Can you work these out from the model? Positions are in its coordinate system, mm. Give positions to 0.01 mm unless a question says otherwise; leave off trailing zeros. Order: outer loops, then holes, each group sorted by start corner. A loop starts at its lowest first (then second) coordinate and runs counter-clockwise, first axis right, second up.
Item 1: I'm going to push a flat-ended pin straight in: pin 1 Ø2.5 at (x, y) = (45, 4) entering from -Z. Where does the tip first touch, or does it pass through?
Item 2: If I drill on line 1 along Z through (x, y) = (-5.5, 0.5); line 2 along Z through (x, y) = (23, 0.5), over which ranges is the centre line in solid material (lowest first)?
Item 3: I want a section at C-C, the plane z = 30.5. Write out the boundary of the cut face in (x, y), then the cut area to 3 significant figures.
Item 4: I want a section at A-A, the plane z = -45.5. Count the separate pieces of the cut face and the enclosed holes in it, then the cut area to 3 significant figures.
Item 5: I want a section at D-D, the plane z = 45.5. Write out the boundary of the cut face in (x, y), then the cut area to 3 significant figures.
Item 6: I want a section at B-B, the plane x = -3. Write out the boundary of the cut face in (y, z), then the cut area to 3 significant figures.
```python
from build123d import *

# Parameters (mm, degrees)
SKETCH1_W                       = 96
SKETCH1_H                       = 96
SKETCH1_W_2                     = 80
SKETCH1_H_2                     = 80
BOSS_EXTRUDE1_DEPTH             = 8
F_3_0_3_DIAMETER_HOLE6_D        = 3
F_3_0_3_DIAMETER_HOLE6_DEPTH    = 7.5
F_3_0_3_DIAMETER_HOLE3_D        = 3
F_3_0_3_DIAMETER_HOLE3_DEPTH    = 7.5
SKETCH27_W                      = 82
SKETCH27_H                      = 82
CUT_EXTRUDE2_DEPTH              = 10
F_3_4_3_4_DIAMETER_HOLE1_D      = 3.4
SKETCH38_W                      = 85
SKETCH38_H                      = 85
CUT_EXTRUDE4_DEPTH              = 10
SKETCH44_W                      = 4
SKETCH44_H                      = 4
BOSS_EXTRUDE2_DEPTH             = 8
SKETCH45_W                      = 4
SKETCH45_H                      = 3.5
BOSS_EXTRUDE3_DEPTH             = 8
TAP_DRILL_FOR_M3X0_5_TAP1_D     = 2.5
SKETCH49_W                      = 96
SKETCH49_H                      = 1.5
CUT_EXTRUDE5_DEPTH              = 146
TAP_DRILL_FOR_M3X0_5_TAP2_D     = 3
TAP_DRILL_FOR_M3X0_5_TAP2_DEPTH = 5.5
TAP_DRILL_FOR_M3X0_5_TAP3_D     = 3
TAP_DRILL_FOR_M3X0_5_TAP3_DEPTH = 5.5
TAP_DRILL_FOR_M3X0_5_TAP4_D     = 3
TAP_DRILL_FOR_M3X0_5_TAP5_D     = 3
TAP_DRILL_FOR_M3X0_5_TAP6_D     = 3
TAP_DRILL_FOR_M3X0_5_TAP6_DEPTH = 5.5


with BuildPart() as part:
    # Sketch1 → Boss-Extrude1 (new body)
    with BuildSketch(Plane(origin=(0, 0, 0), x_dir=(1, 0, 0), z_dir=(0, 1, 0))):
        Rectangle(SKETCH1_W, SKETCH1_H)
        Rectangle(SKETCH1_W_2, SKETCH1_H_2, mode=Mode.SUBTRACT)
    extrude(amount=BOSS_EXTRUDE1_DEPTH)

    # Ø3.0 (3) Diameter Hole6
    with Locations(Plane.XY.offset(48)):
        with Locations((45, 4), (-45, 4)):
            Hole(F_3_0_3_DIAMETER_HOLE6_D / 2, depth=F_3_0_3_DIAMETER_HOLE6_DEPTH)

    # Ø3.0 (3) Diameter Hole3
    with Locations(Plane(origin=(0, 0, -48), x_dir=(-1, 0, 0), z_dir=(0, 0, -1))):
        with Locations((-45, 4), (45, 4)):
            Hole(F_3_0_3_DIAMETER_HOLE3_D / 2, depth=F_3_0_3_DIAMETER_HOLE3_DEPTH)

    # Sketch27 → Cut-Extrude2 (cut)
    with BuildSketch(Plane(origin=(0, 8, 0), x_dir=(1, 0, 0), z_dir=(0, 1, 0))):
        Rectangle(SKETCH27_W, SKETCH27_H)
    extrude(amount=-CUT_EXTRUDE2_DEPTH, mode=Mode.SUBTRACT)

    # Ø3.4 (3.4) Diameter Hole1 (through all)
    with Locations(Plane(origin=(0, 0, 0), x_dir=(-1, 0, 0), z_dir=(0, -1, 0))):
        with Locations((-23, 45.5), (23, 45.5), (45.5, 23), (45.5, -25), (23, -45.5), (-23, -45.5), (-45.5, -25), (-45.5, 25)):
            Hole(F_3_4_3_4_DIAMETER_HOLE1_D / 2)

    # Sketch38 → Cut-Extrude4 (cut)
    with BuildSketch(Plane(origin=(0, 8, 0), x_dir=(1, 0, 0), z_dir=(0, 1, 0))):
        Rectangle(SKETCH38_W, SKETCH38_H)
    extrude(amount=-CUT_EXTRUDE4_DEPTH, mode=Mode.SUBTRACT)

    # Sketch44 → Boss-Extrude2 (add)
    with BuildSketch(Plane.XZ):
        with Locations((40.5, -40.5)):
            Rectangle(SKETCH44_W, SKETCH44_H)
        with Locations((-40.5, -40.5)):
            Rectangle(SKETCH44_W, SKETCH44_H)
        with Locations((-40.5, 40.5)):
            Rectangle(SKETCH44_W, SKETCH44_H)
        with Locations((40.5, 40.5)):
            Rectangle(SKETCH44_W, SKETCH44_H)
    extrude(amount=-BOSS_EXTRUDE2_DEPTH)

    # Sketch45 → Boss-Extrude3 (add)
    with BuildSketch(Plane(origin=(0, 8, 0), x_dir=(1, 0, 0), z_dir=(0, 1, 0))):
        with Locations((-40.5, 36.75)):
            Rectangle(SKETCH45_W, SKETCH45_H)
    extrude(amount=-BOSS_EXTRUDE3_DEPTH)

    # Tap Drill for M3x0.5 Tap1 (through all)
    with Locations(Plane(origin=(0, 8, 0), x_dir=(1, 0, 0), z_dir=(0, 1, 0))):
        with Locations((41.5, 41.5), (41.5, -41.5), (-41.5, -41.5), (-44.05, 37.33)):
            Hole(TAP_DRILL_FOR_M3X0_5_TAP1_D / 2)

    # Sketch49 → Cut-Extrude5 (cut)
    with BuildSketch(Plane(origin=(48, 0, 0), x_dir=(0, 0, -1), z_dir=(1, 0, 0))):
        with Locations((0, 7.25)):
            Rectangle(SKETCH49_W, SKETCH49_H)
    extrude(amount=-CUT_EXTRUDE5_DEPTH, mode=Mode.SUBTRACT)

    # Tap Drill for M3x0.5 Tap2
    with Locations(Plane.ZY.offset(48)):
        with Locations((30.5, 3.7), (-30.5, 3.7)):
            Hole(TAP_DRILL_FOR_M3X0_5_TAP2_D / 2, depth=TAP_DRILL_FOR_M3X0_5_TAP2_DEPTH)

    # Tap Drill for M3x0.5 Tap3
    with Locations(Plane(origin=(0, 0, -48), x_dir=(-1, 0, 0), z_dir=(0, 0, -1))):
        with Locations((30.5, 3.7), (-30.5, 3.7)):
            Hole(TAP_DRILL_FOR_M3X0_5_TAP3_D / 2, depth=TAP_DRILL_FOR_M3X0_5_TAP3_DEPTH)

    # Tap Drill for M3x0.5 Tap4 (through all)
    with Locations(Plane(origin=(48, 0, 0), x_dir=(0, 0, -1), z_dir=(1, 0, 0))):
        with Locations((30.5, 3.7), (-30.5, 3.7)):
            Hole(TAP_DRILL_FOR_M3X0_5_TAP4_D / 2)

    # Tap Drill for M3x0.5 Tap5 (through all)
    with Locations(Plane.XY.offset(48)):
        with Locations((30.5, 3.7), (-30.5, 3.7)):
            Hole(TAP_DRILL_FOR_M3X0_5_TAP5_D / 2)

    # Tap Drill for M3x0.5 Tap6
    with Locations(Plane(origin=(0, 0, -48), x_dir=(-1, 0, 0), z_dir=(0, 0, -1))):
        with Locations((38.1, 3.7), (-38.1, 3.7)):
            Hole(TAP_DRILL_FOR_M3X0_5_TAP6_D / 2, depth=TAP_DRILL_FOR_M3X0_5_TAP6_DEPTH)


solid = part.part
```
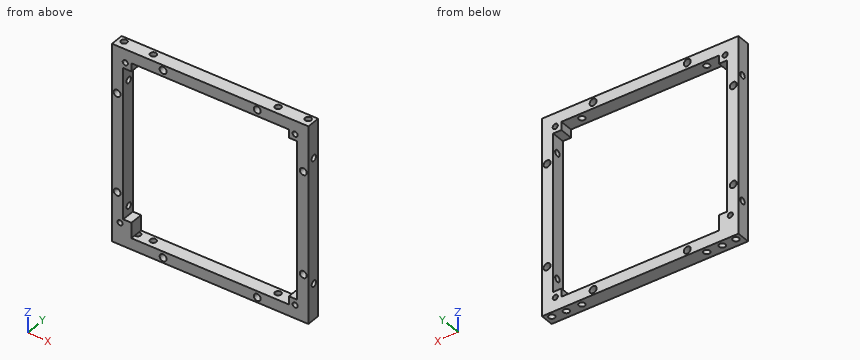
Results list:
1. pin 1: stops at z = -40.5
2. line 1: z = -48 to -42.5, 42.5 to 48
2. line 2: z = -48 to -47.2, -43.8 to -42.5, 42.5 to 43.8, 47.2 to 48
3. outline: (-48, 0) - (-42.5, 0) - (-42.5, 2.2) - (-48, 2.2) - close; (-48, 5.2) - (-42.5, 5.2) - (-42.5, 6.5) - (-48, 6.5) - close; (42.5, 0) - (48, 0) - (48, 2.2) - (42.5, 2.2) - close; (42.5, 5.2) - (48, 5.2) - (48, 6.5) - (42.5, 6.5) - close
3. area: 38.5 mm2
4. separate pieces: 3
4. enclosed holes: 6
4. area: 537 mm2
5. outline: (-48, 0) - (-24.7, 0) - (-24.7, 6.5) - (-48, 6.5) - close; (-21.3, 0) - (21.3, 0) - (21.3, 6.5) - (-21.3, 6.5) - close; (24.7, 0) - (48, 0) - (48, 6.5) - (24.7, 6.5) - close; hole circle Ø3 at (-45, 4); hole circle Ø3 at (-30.5, 3.7); hole circle Ø3 at (30.5, 3.7); hole circle Ø3 at (45, 4)
5. area: 552 mm2
6. outline: (0, -48) - (6.5, -48) - (6.5, -42.5) - (0, -42.5) - close; (0, 42.5) - (6.5, 42.5) - (6.5, 48) - (0, 48) - close
6. area: 71.5 mm2
